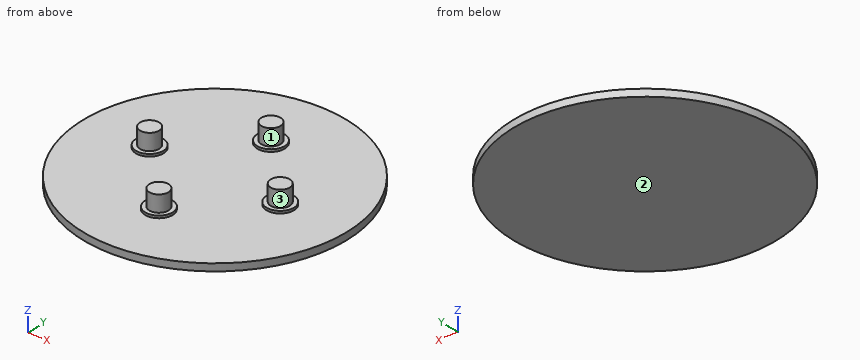
```python
from build123d import *

# Parameters (mm, degrees)
F0_R      = 55
F1_DEPTH  = 3
F2_R      = 5.75
F3_DEPTH  = 1
F5_R      = 4
F6_DEPTH  = 6.8
F4_R      = 4
F7_DEPTH  = 6.8
F8_R      = 4
F9_DEPTH  = 6.8
F10_R     = 4
F11_DEPTH = 6.8


# Not quite as in the source:
# - a feature of the source that left no trace in its solid (it failed there, or was rolled back) is left out


with BuildPart() as f1:
    # F0 (on Top) → F1 (new body)
    with BuildSketch(Plane.XY):
        Circle(F0_R)
    extrude(amount=F1_DEPTH)

    # F2 (on face) → F3 (join)
    with BuildSketch(Plane.XY.offset(3)):
        with Locations((-27.5, 0)):
            Circle(F2_R)
        with Locations((27.5, 0)):
            Circle(F2_R)
        with Locations((0, 27.5)):
            Circle(F2_R)
        with Locations((0, -27.5)):
            Circle(F2_R)
    extrude(amount=F3_DEPTH)

    # F5 (on face) → F6 (join)
    with BuildSketch(Plane.XY.offset(4)):
        with Locations((27.5, 0)):
            Circle(F5_R)
    extrude(amount=F6_DEPTH)

    # F4 (on face) → F7 (join)
    with BuildSketch(Plane.XY.offset(4)):
        with Locations((-27.5, 0)):
            Circle(F4_R)
    extrude(amount=F7_DEPTH)

    # F8 (on face) → F9 (join)
    with BuildSketch(Plane.XY.offset(4)):
        with Locations((0, 27.5)):
            Circle(F8_R)
    extrude(amount=F9_DEPTH)

    # F10 (on face) → F11 (join)
    with BuildSketch(Plane.XY.offset(4)):
        with Locations((0, -27.5)):
            Circle(F10_R)
    extrude(amount=F11_DEPTH)


solid = f1.part
```
Geometry check sheet. Reference: the model listing, model coordinates, mm. Face numbers are marked on the shaded views. Coordinates: 2 decimals unless noted, no trailing zeros. Loops run counter-clockwise (first coordinate to the right, second up) from the corner with the lowest first, then second, coordinate; pieces in that order, holes last.
Item 1: Thickness scan on line 1 (Z direction, x = -31, y = 22); line 2 (Y direction, x = -2, z = 7.75); line 3 (X direction, y = 30.5, z = 8.75). Record the ranges inside material, lowest first.
Item 2: Release check for a two-part mould opening along Y. For the marked faces 1, 2 and 3 record: released by +Y, released by -Y, zero draft, split by the parting line, or undercut.
Item 3: Go/stop test with flat-tipped pins: pin 1 Ø8 at (x, y) = (36.5, -18.5) entering from +Z; pin 2 Ø1.5 at (y, z) = (-31, 1.5) entering from +X; pin 3 Ø1.5 at (y, z) = (-26.5, 8.5) entering from +X. Record where each tip stops, or that it passes through.
Item 4: Sectioned sample at D-D, the plane x = -27.5. Record the boundary of the cut face in (y, z), then the cut area to 3 significant figures.
Item 5: Sectioned sample at B-B, the plane z = 6. Record the boundary of the cut face in (x, y), then the cut area to 3 significant figures.
Item 6: Sectioned sample at A-A, the plane x = 0. Record the boundary of the cut face in (y, z).
Check result:
1. line 1: z = 0 to 3
1. line 2: y = -30.96 to -24.04, 24.04 to 30.96
1. line 3: x = -2.65 to 2.65
2. face 1: undercut
2. face 2: zero draft
2. face 3: split by the parting line
3. pin 1: stops at z = 3
3. pin 2: stops at x = 45.93
3. pin 3: stops at x = 3.99
4. outline: (-47.63, 0) - (47.63, 0) - (47.63, 3) - (5.75, 3) - (5.75, 4) - (4, 4) - (4, 10.8) - (-4, 10.8) - (-4, 4) - (-5.75, 4) - (-5.75, 3) - (-47.63, 3) - close
4. area: 352 mm2
5. outline: circle Ø8 at (-27.5, 0); circle Ø8 at (0, -27.5); circle Ø8 at (0, 27.5); circle Ø8 at (27.5, 0)
5. area: 201 mm2
6. outline: (-55, 0) - (55, 0) - (55, 3) - (33.25, 3) - (33.25, 4) - (31.5, 4) - (31.5, 10.8) - (23.5, 10.8) - (23.5, 4) - (21.75, 4) - (21.75, 3) - (-21.75, 3) - (-21.75, 4) - (-23.5, 4) - (-23.5, 10.8) - (-31.5, 10.8) - (-31.5, 4) - (-33.25, 4) - (-33.25, 3) - (-55, 3) - close
